Work out the finished part from the listing and answer in its coordinate system (mm). Face numbers are marked on the shaded views. A direction names the side the tool comes from. Give positions to 0.01 mm unless a question says otherwise; leave off trailing zeros. Write each loop counter-clockwise with the first axis right and the second up, starting at its lowest first coordinate (ties: lowest second). Pieces come first, ordered by that corner, then holes. Notation, with made-up numbers: (27.5, 59) - (40.5, 59) arc R18 ccw to (40.5, 79) - close; hole circle Ø6 at (33, -1.75). An arc over 180 degrees is marked (long way). Write each question's results on one line, items separated by ' | '. Start each with the question number.
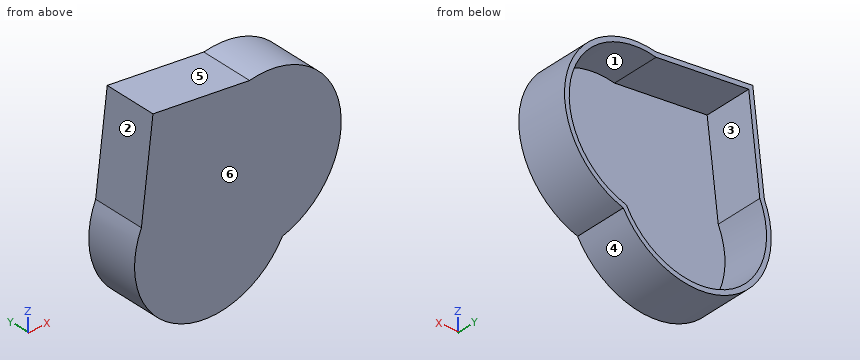
from build123d import *

# Parameters (mm, degrees)
F1_DEPTH = 27.686
F3_T     = -2.54


with BuildPart() as f1:
    # F0 (on Front) → F1 (new body)
    with BuildSketch(Plane.XZ):
        with BuildLine():
            Line((32.9105183482, -44.3405173719), (-37.6401729882, 47.4936179817))
            Line((-37.6401729882, 47.4936179817), (-43.9463816583, -5.3208619356))
            ThreePointArc((-43.9463816583, -5.3208619356), (-24.0622741562, -61.3574262782), (32.9105183482, -44.3405173719))
        make_face()
    extrude(amount=F1_DEPTH)

    # F2: F1 across face


with BuildPart() as f1_1:
    add(f1.part)
    add(f1.part.mirror(Plane(origin=(-2.36482732, -13.843, 1.5765503049), x_dir=(0, 1, 0), z_dir=(0.7930033869, 0, 0.6092172259))))

    # F3
    f3_openings = [f1_1.faces().sort_by_distance(p)[0] for p in [
        (4.890948, 0, -7.868117),
    ]]
    offset(amount=F3_T, openings=f3_openings, kind=Kind.INTERSECTION)


solid = f1_1.part
Q1. Given pin 1 (4 mm diameter, centred on x = 44, z = -22, fed in from +Y); pin 2 (10 mm diameter, centred on x = 36, y = -23, fed in from +Z); pin 3 (2 mm diameter, centred on y = -24, z = -36.5, fed in from +X), each flat-ended and moving along its own axis, determine where each tip first touches the part or whether it passes through.
Q2. The mould has two halves that part along Z. Classify the marked faces 3, 4, 5 and 6: pulls with the +Z half, pulls with the -Z half, needs draft (parallel to the pull), parting line crosses it, or undercut.
Q3. A tool of negligible diameter and unlimited length cuts with its end or side. For the marked faces 1 and 2, from which of +Z, -Z, +X, -X, +Y, -Y can it reach the whole face along a straight path? Write none if from no direction.
Q4. A cutting plane is placed at C-C, the plane x = 28.5. Write down the section's boundary in (y, z), and give its area (3 significant figures).
Q5. Consider L1, parallel to Y at x = 19.5, z = -2; L2, parallel to Z at x = 14.5, y = -2; L3, parallel to Z at x = 41.5, y = -8. Determine where each line is inside the solid, lowest interval first.
Q6. A cutting plane is placed at A-A, the plane y = -17. Write down the section's boundary in (x, z), and give its area (3 significant figures).
Q7. A cutting plane is placed at B-B, the plane z = 27. Write down the section's boundary in (x, y).
Result:
1) pin 1: stops at y = -25.15 | pin 2: stops at z = 39.53 | pin 3: stops at x = 49.79
2) face 3: undercut | face 4: parting line crosses it | face 5: pulls with the +Z half | face 6: needs draft
3) face 1: +Y | face 2: +Z, -X, +Y, -Y
4) outline: (-27.69, -50.65) - (0, -50.65) - (0, -46.51) - (-25.15, -46.51) - (-25.15, 37.42) - (0, 37.42) - (0, 40) - (-27.69, 40) - close | area: 399 mm2
5) L1: y = -27.69 to -25.15 | L2: z = -61.61 to -58.76, 37.48 to 40.05 | L3: z = -41.04 to -38.16, 32.89 to 35.77
6) outline: (-43.95, -5.32) arc R43.15 ccw to (32.91, -44.34) arc R43.15 ccw to (15.02, 39.98) - (-37.64, 47.49) - close; hole (-41.47, -6.01) arc R40.61 ccw to (31.22, -42.15) arc R40.61 ccw to (15.04, 37.41) - (-35.43, 44.61) - close | area: 915 mm2
7) outline: (-40.09, -27.69) - (53.19, -27.69) - (53.19, 0) - (49.59, 0) - (49.59, -25.15) - (-37.53, -25.15) - (-37.53, 0) - (-40.09, 0) - close
